The listing builds one solid part. Answer for the finished solid, in the listing's coordinates (mm). Give positions to 0.01 mm unless a question says otherwise; leave off trailing zeros. Order: outer loops, then holes, each group sorted by start corner. A loop starts at its lowest first (then second) coordinate and runs counter-clockwise, first axis right, second up.
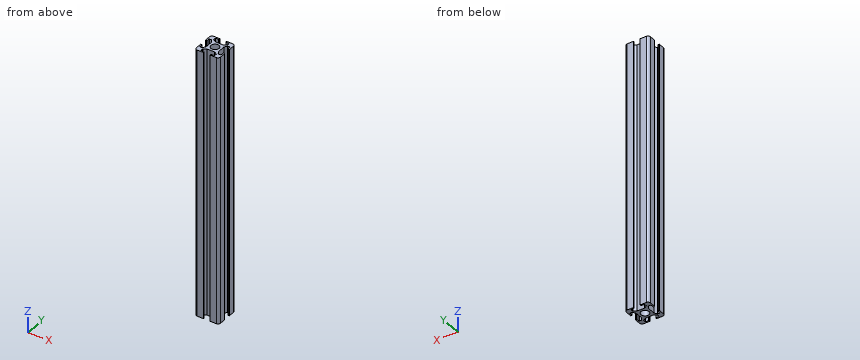
```python
from build123d import *

# Parameters (mm, degrees)
CROQUIS1_R              = 5.85
SALIENTE_EXTRUIR1_DEPTH = 390


with BuildPart() as part:
    # Croquis1 → Saliente-Extruir1 (new body)
    with BuildSketch(Plane.XY):
        with BuildLine():
            Line((-17.5, -5), (-16, -5))
            ThreePointArc((-16, -5), (-15.646446609, -5.146446609), (-15.5, -5.5))
            Line((-15.5, -5.5), (-15.5, -9.5))
            ThreePointArc((-15.5, -9.5), (-15.353553391, -9.853553391), (-15, -10))
            Line((-15, -10), (-11.790147321, -10))
            ThreePointArc((-11.790147321, -10), (-11.539192936, -9.932460283), (-11.356036103, -9.748087586))
            Line((-11.356036103, -9.748087586), (-9.065888782, -5.740718013))
            ThreePointArc((-9.065888782, -5.740718013), (-9.016752854, -5.620974478), (-9, -5.492630427))
            Line((-9, -5.492630427), (-9, 5.492630427))
            ThreePointArc((-9, 5.492630427), (-9.016752854, 5.620974478), (-9.065888782, 5.740718013))
            Line((-9.065888782, 5.740718013), (-11.356036103, 9.748087586))
            ThreePointArc((-11.356036103, 9.748087586), (-11.539192936, 9.932460283), (-11.790147321, 10))
            Line((-11.790147321, 10), (-15, 10))
            ThreePointArc((-15, 10), (-15.353553391, 9.853553391), (-15.5, 9.5))
            Line((-15.5, 9.5), (-15.5, 5.5))
            ThreePointArc((-15.5, 5.5), (-15.646446609, 5.146446609), (-16, 5))
            Line((-16, 5), (-17.5, 5))
            Line((-17.5, 5), (-17.5, 14))
            ThreePointArc((-17.5, 14), (-16.474873734, 16.474873734), (-14, 17.5))
            Line((-14, 17.5), (-5, 17.5))
            Line((-5, 17.5), (-5, 16))
            ThreePointArc((-5, 16), (-5.146446609, 15.646446609), (-5.5, 15.5))
            Line((-5.5, 15.5), (-9.5, 15.5))
            ThreePointArc((-9.5, 15.5), (-9.853553391, 15.353553391), (-10, 15))
            Line((-10, 15), (-10, 11.790147321))
            ThreePointArc((-10, 11.790147321), (-9.932460283, 11.539192936), (-9.748087586, 11.356036103))
            Line((-9.748087586, 11.356036103), (-5.740718013, 9.065888782))
            ThreePointArc((-5.740718013, 9.065888782), (-5.620974478, 9.016752854), (-5.492630427, 9))
            Line((-5.492630427, 9), (5.492630427, 9))
            ThreePointArc((5.492630427, 9), (5.620974478, 9.016752854), (5.740718013, 9.065888782))
            Line((5.740718013, 9.065888782), (9.748087586, 11.356036103))
            ThreePointArc((9.748087586, 11.356036103), (9.932460283, 11.539192936), (10, 11.790147321))
            Line((10, 11.790147321), (10, 15))
            ThreePointArc((10, 15), (9.853553391, 15.353553391), (9.5, 15.5))
            Line((9.5, 15.5), (5.5, 15.5))
            ThreePointArc((5.5, 15.5), (5.146446609, 15.646446609), (5, 16))
            Line((5, 16), (5, 17.5))
            Line((5, 17.5), (14, 17.5))
            ThreePointArc((14, 17.5), (16.474873734, 16.474873734), (17.5, 14))
            Line((17.5, 14), (17.5, 5))
            Line((17.5, 5), (16, 5))
            ThreePointArc((16, 5), (15.646446609, 5.146446609), (15.5, 5.5))
            Line((15.5, 5.5), (15.5, 9.5))
            ThreePointArc((15.5, 9.5), (15.353553391, 9.853553391), (15, 10))
            Line((15, 10), (11.790147321, 10))
            ThreePointArc((11.790147321, 10), (11.539192936, 9.932460283), (11.356036103, 9.748087586))
            Line((11.356036103, 9.748087586), (9.065888782, 5.740718013))
            ThreePointArc((9.065888782, 5.740718013), (9.016752854, 5.620974478), (9, 5.492630427))
            Line((9, 5.492630427), (9, -5.492630427))
            ThreePointArc((9, -5.492630427), (9.016752854, -5.620974478), (9.065888782, -5.740718013))
            Line((9.065888782, -5.740718013), (11.356036103, -9.748087586))
            ThreePointArc((11.356036103, -9.748087586), (11.539192936, -9.932460283), (11.790147321, -10))
            Line((11.790147321, -10), (15, -10))
            ThreePointArc((15, -10), (15.353553391, -9.853553391), (15.5, -9.5))
            Line((15.5, -9.5), (15.5, -5.5))
            ThreePointArc((15.5, -5.5), (15.646446609, -5.146446609), (16, -5))
            Line((16, -5), (17.5, -5))
            Line((17.5, -5), (17.5, -14))
            ThreePointArc((17.5, -14), (16.474873734, -16.474873734), (14, -17.5))
            Line((14, -17.5), (5, -17.5))
            Line((5, -17.5), (5, -16))
            ThreePointArc((5, -16), (5.146446609, -15.646446609), (5.5, -15.5))
            Line((5.5, -15.5), (9.5, -15.5))
            ThreePointArc((9.5, -15.5), (9.853553391, -15.353553391), (10, -15))
            Line((10, -15), (10, -11.790147321))
            ThreePointArc((10, -11.790147321), (9.932460283, -11.539192936), (9.748087586, -11.356036103))
            Line((9.748087586, -11.356036103), (5.740718013, -9.065888782))
            ThreePointArc((5.740718013, -9.065888782), (5.620974478, -9.016752854), (5.492630427, -9))
            Line((5.492630427, -9), (-5.492630427, -9))
            ThreePointArc((-5.492630427, -9), (-5.620974478, -9.016752854), (-5.740718013, -9.065888782))
            Line((-5.740718013, -9.065888782), (-9.748087586, -11.356036103))
            ThreePointArc((-9.748087586, -11.356036103), (-9.932460283, -11.539192936), (-10, -11.790147321))
            Line((-10, -11.790147321), (-10, -15))
            ThreePointArc((-10, -15), (-9.853553391, -15.353553391), (-9.5, -15.5))
            Line((-9.5, -15.5), (-5.5, -15.5))
            ThreePointArc((-5.5, -15.5), (-5.146446609, -15.646446609), (-5, -16))
            Line((-5, -16), (-5, -17.5))
            Line((-5, -17.5), (-14, -17.5))
            ThreePointArc((-14, -17.5), (-16.474873734, -16.474873734), (-17.5, -14))
            Line((-17.5, -14), (-17.5, -5))
        make_face()
        Circle(CROQUIS1_R, mode=Mode.SUBTRACT)
    extrude(amount=SALIENTE_EXTRUIR1_DEPTH)


solid = part.part
```
1) Given P1, Ø0.8, axis at y = -16.5, z = 193.5, coming from the +X side; P2, Ø1.6, axis at y = 17, z = 177, coming from the -X side; P3, Ø0.8, axis at x = 17, z = 104.5, coming from the +Y side; P4, Ø8, axis at x = -1.5, z = 46, coming from the -Y side, each flat-ended and moving along its own axis, determine where each tip first touches the part or whether it passes through.
Geometry says:
P1: stops at x = 16.8
P2: stops at x = -16.72
P3: stops at y = 16.34
P4: stops at y = -17.5
2) Find section A-A (x = 0). Write down the section's boundary in (y, z).
Geometry says:
outline: (-9, 0) - (-5.85, 0) - (-5.85, 390) - (-9, 390) - close; (5.85, 0) - (9, 0) - (9, 390) - (5.85, 390) - close
3) Straight lines are drawn through the part: probe 1 along Y at (x, z) = (-6.5, 104); probe 2 along Y at (x, z) = (7, 372); probe 3 along Y at (x, z) = (11, 209.5). For each, find the intervals that lie inside material, in ascending order.
Geometry says:
probe 1: y = -17.5 to -15.5, -9.5 to 9.5, 15.5 to 17.5
probe 2: y = -17.5 to -15.5, -9.79 to 9.79, 15.5 to 17.5
probe 3: y = -17.5 to -9.13, 9.13 to 17.5
